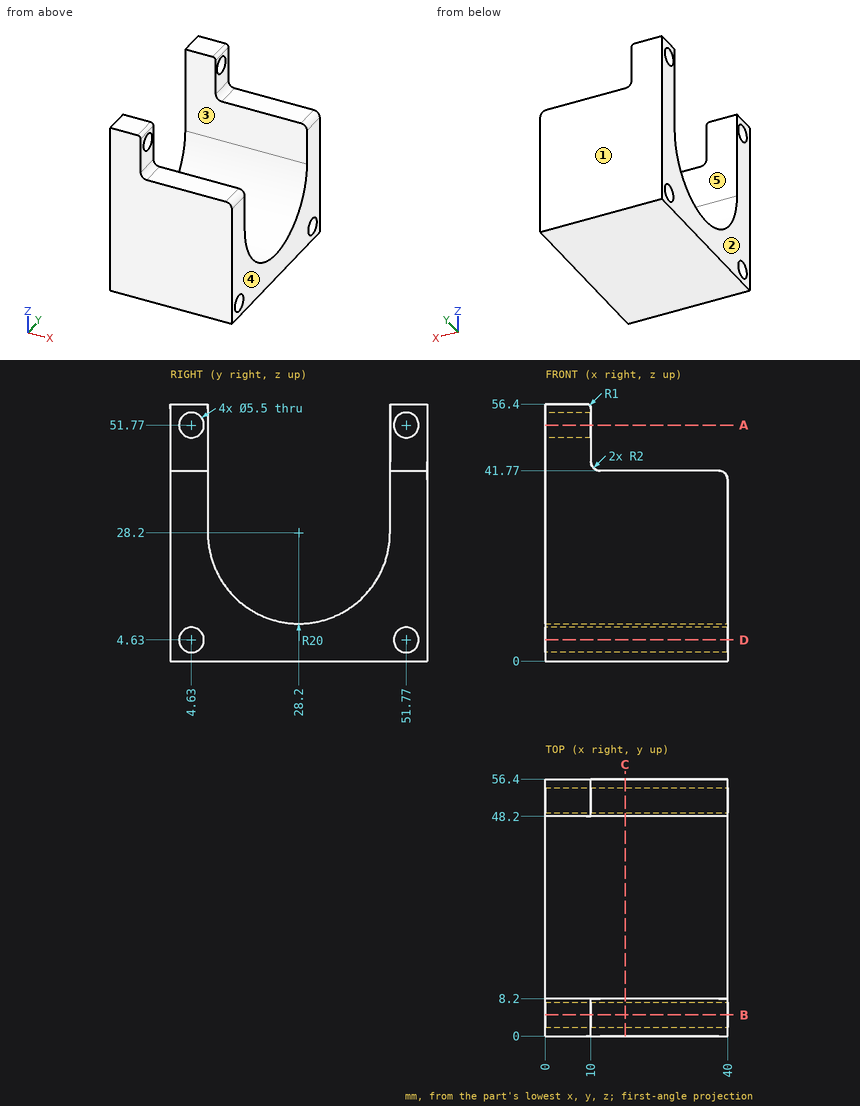
Part print with two shaded views. Sizes in mm from the minimum x, y, z corner. A direction names the side the tool comes from. Round coordinates to 2 decimals unless told otherwise and drop trailing zeros. Order: outer loops, then holes, each group sorted by start corner. A loop starts at its lowest first (then second) coordinate and runs counter-clockwise, first axis right, second up.
(1) Band-saw the part on B-B (y = 4.63). List the corners of the cut face in (x, z), then the cut area to 3 significant figures.
(2) Band-saw the part on C-C (x = 17.5). List the corners of the cut face in (y, z).
(3) Drill centre lines: line 1 (Y direction, x = 7, z = 51.77); line 2 (Y direction, x = 30, z = 4.63); line 3 (Y direction, x = 15, z = 31). Where is each one in solid material? Low to high.
(4) Pin check, flat tips, straight feed: pin 1 (6.5 mm diameter, centred on x = 27.5, y = 5.5, fed in from +Z); pin 2 (9 mm diameter, centred on y = 51.77, z = 51.77, fed in from +X); pin 3 (1 mm diameter, centred on x = 24, y = 25, fed in from +Z). Stop position of each tip, or through.
(5) Pull direction Y, two halves, no side cores. Call the marked faces 1, 2 and 3: released by +Y, released by -Y, zero draft, split by the parting line, or undercut.
(6) 3-axis set-ups, long thin cutter, end or side, ignore diameter. For the marked faces 4 and 5: which of +Z, -Z, +X, -X, +Y, -Y reach the whole face in a straight line?
(7) Band-saw the part on D-D (z = 4.63). List the corners of the cut face in (x, y), then the cut area to 3 significant figures.
(8) Band-saw the part on A-A (z = 51.77). List the corners of the cut face in (x, y), then the cut area to 3 significant figures.
Verdict:
1. outline: (0, 0) - (40, 0) - (40, 1.88) - (0, 1.88) - close; (0, 7.38) - (40, 7.38) - (40, 39.77) arc R2 ccw to (38, 41.77) - (12, 41.77) arc R2 cw to (10, 43.77) - (10, 49.02) - (0, 49.02) - close; (0, 54.52) - (10, 54.52) - (10, 55.4) arc R1 ccw to (9, 56.4) - (0, 56.4) - close
1. area: 1,540 mm2
2. outline: (0, 0) - (56.4, 0) - (56.4, 41.77) - (48.2, 41.77) - (48.2, 28.2) arc R20 cw to (8.2, 28.2) - (8.2, 41.77) - (0, 41.77) - close; hole circle Ø5.5 at (4.63, 4.63); hole circle Ø5.5 at (51.77, 4.63)
3. line 1: y = 0 to 1.88, 7.38 to 8.2, 48.2 to 49.02, 54.52 to 56.4
3. line 2: y = 0 to 1.88, 7.38 to 49.02, 54.52 to 56.4
3. line 3: y = 0 to 8.2, 48.2 to 56.4
4. pin 1: stops at z = 41.77
4. pin 2: stops at x = 10
4. pin 3: stops at z = 8.55
5. face 1: released by +Y
5. face 2: zero draft
5. face 3: undercut
6. face 4: +Z, -Z, +X, +Y, -Y
6. face 5: +Z, +X, -X
7. outline: (0, 0) - (40, 0) - (40, 1.88) - (0, 1.88) - close; (0, 7.38) - (40, 7.38) - (40, 49.02) - (0, 49.02) - close; (0, 54.52) - (40, 54.52) - (40, 56.4) - (0, 56.4) - close
7. area: 1,820 mm2
8. outline: (0, 0) - (10, 0) - (10, 1.88) - (0, 1.88) - close; (0, 7.38) - (10, 7.38) - (10, 8.2) - (0, 8.2) - close; (0, 48.2) - (10, 48.2) - (10, 49.02) - (0, 49.02) - close; (0, 54.52) - (10, 54.52) - (10, 56.4) - (0, 56.4) - close
8. area: 54.0 mm2
